The figure shows three views and two pictorial views of one solid part (mm, origin at its lowest corner). Answer the questions. A direction names the side the tool comes from. Round coordinates to 2 decimals unless told otherwise and drop trailing zeros. Loops run counter-clockwise (first coordinate to the right, second up) from the corner with the lowest first, then second, coordinate; pieces in that order, holes last. Notation, with made-up numbers: (-5.5, -23) -> (41.5, -23) arc R22 cw to (41.5, -6) -> close; hole circle Ø11 at (59.25, -31). An arc over 180 degrees is marked (long way). Put each result on its own line as item: value.
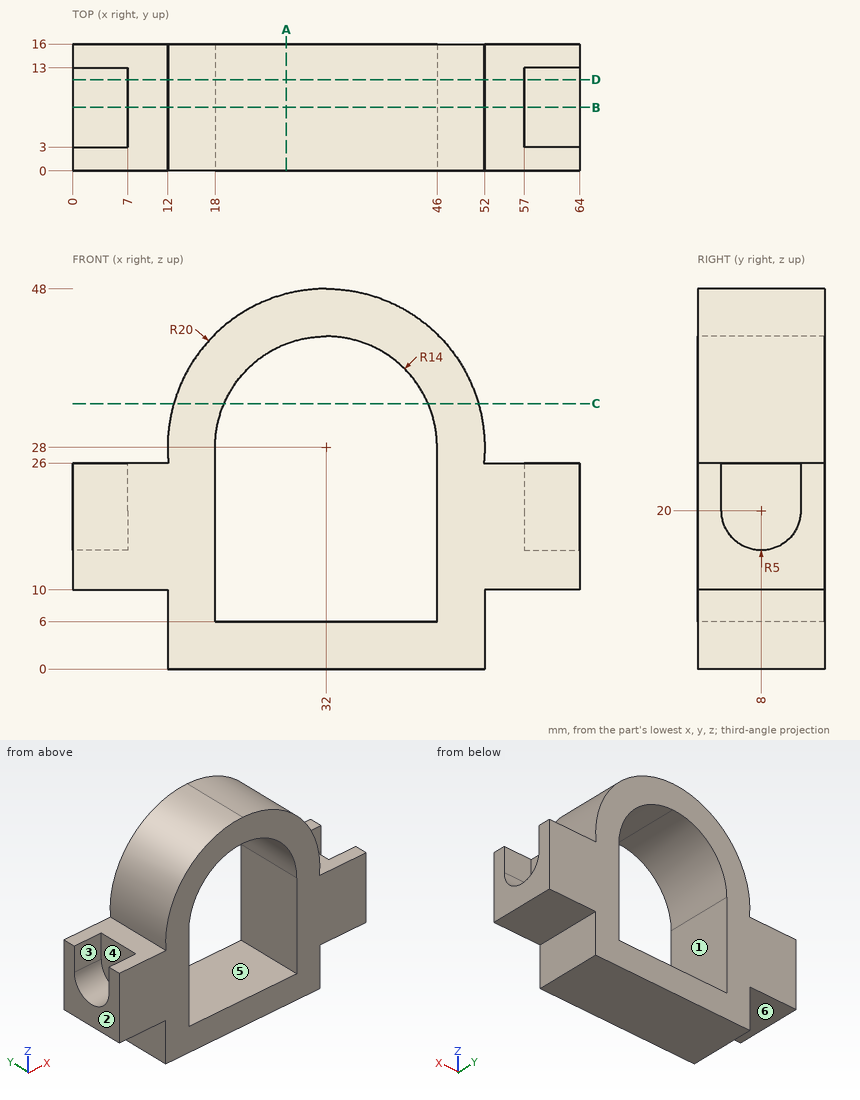
Item 1: Which of the six approach directions +Z, -Z, +X, -X, +Y, -Y give full straight-line access (tool end or side, diameter ignored) to the marked faces 4, 5 and 6?
Derived:
face 4: +Z, -X
face 5: +Y, -Y
face 6: -Z, -X, +Y, -Y
Item 2: The part is cut by section C-C (z = 33.5). Determine the outline of the cut face in (x, y).
Derived:
outline: (12.77, 0) -> (19.13, 0) -> (19.13, 16) -> (12.77, 16) -> close; (44.87, 0) -> (51.23, 0) -> (51.23, 16) -> (44.87, 16) -> close
Item 3: The part is cut by section D-D (y = 11.5). Determine the outline of the cut face in (x, z).
Derived:
outline: (0, 10) -> (12, 10) -> (12, 0) -> (52, 0) -> (52, 10) -> (64, 10) -> (64, 16.43) -> (57, 16.43) -> (57, 26) -> (51.9, 26) arc R20 ccw (long way) to (12.1, 26) -> (7, 26) -> (7, 16.43) -> (0, 16.43) -> close; hole (18, 6) -> (46, 6) -> (46, 28) arc R14 ccw to (18, 28) -> close
Item 4: Flat-ended cylindrical pins translate along their axes: pin 1 Ø3.5 at (x, y) = (3.5, 9.5) entering from -Z; pin 2 Ø8 at (x, z) = (52.5, 40) entering from -Y; pin 3 Ø5 at (y, z) = (8, 19) entering from +X; pin 4 Ø9.5 at (x, y) = (7, 10) entering from +Z. Find the tip coordinate at first contact, or state that the pin passes through.
Derived:
pin 1: stops at z = 10
pin 2: stops at y = 0
pin 3: stops at x = 57
pin 4: stops at z = 26
Item 5: The part is cut by section B-B (y = 8). Determine the outline of the cut face in (x, z), then the cut area to 3 significant figures.
Derived:
outline: (0, 10) -> (12, 10) -> (12, 0) -> (52, 0) -> (52, 10) -> (64, 10) -> (64, 15) -> (57, 15) -> (57, 26) -> (51.9, 26) arc R20 ccw (long way) to (12.1, 26) -> (7, 26) -> (7, 15) -> (0, 15) -> close; hole (18, 6) -> (46, 6) -> (46, 28) arc R14 ccw to (18, 28) -> close
area: 1,050 mm^2
Item 6: Find the intervals of material crossed by line 1 along X through (y, z) = (7.5, 28); line 2 along X through (y, z) = (14.5, 25.5); line 3 along Z through (x, y) = (32, 9), in increasing order.
Derived:
line 1: x = 12 to 18, 46 to 52
line 2: x = 0 to 18, 46 to 64
line 3: z = 0 to 6, 42 to 48
Item 7: For a pull along X with two mould halves and no side action, classify the marked faces 1, 2 and 3 as pulls with the +X half, pulls with the -X half, needs draft (parallel to the pull), parting line crosses it, or undercut.
Derived:
face 1: undercut
face 2: pulls with the -X half
face 3: needs draft
Item 8: The part is cut by section A-A (x = 27). Determine the outline of the cut face in (y, z).
Derived:
outline: (0, 0) -> (16, 0) -> (16, 6) -> (0, 6) -> close; (0, 41.08) -> (16, 41.08) -> (16, 47.36) -> (0, 47.36) -> close
